Geometry: final body of the model. Coordinates: model frame, mm. A direction names the side the tool comes from. Coordinates: 2 decimals unless noted, no trailing zeros. Write each loop counter-clockwise with the first axis right and the second up, starting at its lowest first coordinate (ties: lowest second). Pieces come first, ordered by that corner, then holes.
from build123d import *

# Parameters (mm, degrees)
EXTRUDE_1_DEPTH = 2
FILLET_1_R      = 1


with BuildPart() as part:
    # 草图1 → 凸台-拉伸1 (new body)
    with BuildSketch(Plane.XY):
        Polygon((0, 38.932825237), (4, 38.932825237), (4, 37.482825237), (7.2, 37.482825237), (7.2, 38.932825237), (10.4, 38.932825237), (10.4, 43.032825237), (7.2, 43.032825237), (7.2, 44.482825237), (4, 44.482825237), (4, 43.032825237), (0, 43.032825237), (0, 47.532825237), (16.125183107, 47.532825237), (16.125183107, -46.217174763), (0, -46.217174763), (0, -41.717174763), (4, -41.717174763), (4, -43.167174763), (7.2, -43.167174763), (7.2, -41.717174763), (10.4, -41.717174763), (10.4, -37.617174763), (7.2, -37.617174763), (7.2, -36.167174763), (4, -36.167174763), (4, -37.617174763), (0, -37.617174763), (0, -28.667174763), (-4, -28.667174763), (-4, -20.667174763), (0, -20.667174763), (0, -11.717174763), (4, -11.717174763), (4, -13.167174763), (7.2, -13.167174763), (7.2, -11.717174763), (10.4, -11.717174763), (10.4, -7.617174763), (7.2, -7.617174763), (7.2, -6.167174763), (4, -6.167174763), (4, -7.617174763), (0, -7.617174763), (0, 21.982825237), (-4, 21.982825237), (-4, 29.982825237), (0, 29.982825237), align=None)
    extrude(amount=EXTRUDE_1_DEPTH)

    # 圆角1
    fillet_1_edges = [part.edges().sort_by_distance(p)[0] for p in [
        (-4, 29.982825237, 1),
        (-4, 21.982825237, 1),
        (-4, -20.667174763, 1),
        (-4, -28.667174763, 1),
    ]]
    fillet(fillet_1_edges, radius=FILLET_1_R)


solid = part.part
Item 1: Pull-direction query (Y, two-part tool) for faces 4 (the flat face through (0, -16, 1)), 5 (the flat face through (0, -44, 1)), 6 (the flat face through (8, -46.217, 1)); classes: released by +Y, released by -Y, zero draft, split by the parting line, or undercut.
Derived:
face 4: undercut
face 5: zero draft
face 6: released by -Y
Item 2: Section C-C, the plane y = 40.5. Output: boundary loops of the cut face in (x, z), plus the area to 3 significant figures.
Derived:
outline: (10.4, 0) - (16.13, 0) - (16.13, 2) - (10.4, 2) - close
area: 11.5 mm2
Item 3: Section A-A, the plane x = -1.25. Output: boundary loops of the cut face in (y, z).
Derived:
outline: (-28.67, 0) - (-20.67, 0) - (-20.67, 2) - (-28.67, 2) - close; (21.98, 0) - (29.98, 0) - (29.98, 2) - (21.98, 2) - close
Item 4: Section B-B, the plane x = 2.5. Output: boundary loops of the cut face in (y, z).
Derived:
outline: (-46.22, 0) - (-41.72, 0) - (-41.72, 2) - (-46.22, 2) - close; (-37.62, 0) - (-11.72, 0) - (-11.72, 2) - (-37.62, 2) - close; (-7.62, 0) - (38.93, 0) - (38.93, 2) - (-7.62, 2) - close; (43.03, 0) - (47.53, 0) - (47.53, 2) - (43.03, 2) - close
Item 5: Set-up query: faces 1 (the flat face through (0, 45, 1)), 2 (the flat face through (9, -37.617, 1)), 3 (the flat face through (7.2, 38, 1)). Return all of +Z, -Z, +X, -X, +Y, -Y with unobstructed straight access to the full face (end or side cutting, diameter ignored); none if empty.
Derived:
face 1: +Z, -Z, -X, +Y
face 2: +Z, -Z, -X
face 3: +Z, -Z
Item 6: Pin query (flat end, axial travel): pin 1 (1 mm diameter, centred on y = -34, z = 1, fed in from -X). Return the tip coordinate at first contact, or that it passes through.
Derived:
pin 1: stops at x = 0
Item 7: Section D-D, the plane y = 5. Output: boundary loops of the cut face in (x, z), plus the area to 3 significant figures.
Derived:
outline: (0, 0) - (16.13, 0) - (16.13, 2) - (0, 2) - close
area: 32.3 mm2
Item 8: Material intervals for probe 1 along Y at (x, z) = (5, 1.3); probe 2 along Y at (x, z) = (2.5, 0.85); probe 3 along X at (y, z) = (44, 1.7), sorted ascending.
Derived:
probe 1: y = -46.22 to -43.17, -36.17 to -13.17, -6.17 to 37.48, 44.48 to 47.53
probe 2: y = -46.22 to -41.72, -37.62 to -11.72, -7.62 to 38.93, 43.03 to 47.53
probe 3: x = 0 to 4, 7.2 to 16.13
